The model under review builds one solid part; all positions refer to its coordinate system, in mm. A direction names the side the tool comes from. Round coordinates to 2 decimals unless told otherwise and drop trailing zeros. Write each loop counter-clockwise with the first axis right and the second up, starting at its lowest first coordinate (ties: lowest second). Pieces come first, ordered by that corner, then holes. Notation, with made-up numbers: (46, -40) - (72, -40) arc R14 cw to (72, -21) - close; hole circle Ø6 at (42.5, 66). An arc over 180 degrees is marked (long way). Use one line per item in the form item = value.
Autodesk Inventor part; units mm, degrees
ref_plane "Work Plane1" through (29, 0, 0) normal (0, -1, 0) x (1, 0, 0)
ref_plane "YZ Plane" through (0, 0, 0) normal (1, 0, 0) x (0, 1, 0)
ref_plane "XZ Plane" through (0, 0, 0) normal (0, 1, 0) x (-1, 0, 0)
sketch "Sketch1" plane through (0, 0, 0) normal (0, 0, 1) x (1, 0, 0)
  line L0 (0.2709, 0) -> (19.05, 0)
  line L1 (19.05, 0) -> (19.05, 2.413)
  line L2 (19.05, 2.413) -> (2.1084, 2.413)
  line L3 (2.1084, 2.413) -> (0.0001, 2.413)
  line L4 (0.0001, 2.413) -> (0, 2.413)
  line L5 (0, 2.413) -> (0, 4.5847)
  line L6 (0, 4.5847) -> (-2.5654, 4.5847)
  line L7 (-2.5654, 4.5847) -> (-2.5654, 1.8331)
  line L8 (-2.5654, 1.8331) -> (-0.7874, 1.8331)
  line L9 (-0.7874, 1.8331) -> (0.2709, 0)
  line L10 (-6.8885, 0) -> (23.3731, 0)
  line L11 (0, -0.9169) -> (0, 5.5016)
  line L12 (2.1084, 2.413) -> (0, 2.413) construction
  dimension "d1" = 16.9416
  dimension "d2" = 2.1083
  dimension "d3" = 2.5654
  dimension "d4" = 1.778
  dimension "d5" = 60
  dimension "d6" = 4.826
  dimension "d7" = 4.826
  dimension "d8" = 3.6662
  dimension "d9" = 9.1694
  dimension "d26" = 19.05
revolve "Body" add sketch "Sketch1" angle 360 about axis through (0.2709, 0, 0) along (1, 0, 0) contours L9 L11 L3 L2 L1 L0 | L9 L8 L7 L6 L5 L11
sketch "Sketch2" plane through (-2.5654, 0, 0) normal (-1, 0, 0) x (0, 0, 1)
  circle A0 centre (0, 0) radius 1.8331
  line L0 (0, -6.4186) -> (0, 6.4186)
  line L1 (-6.4186, 0) -> (6.4186, 0)
  line L2 (1.8331, 0) -> (0.9165, -1.5875)
  line L3 (0.9165, -1.5875) -> (-0.9165, -1.5875)
  line L4 (-0.9165, -1.5875) -> (-1.8331, 0)
  line L5 (-1.8331, 0) -> (-0.9165, 1.5875)
  line L6 (-0.9165, 1.5875) -> (0.9165, 1.5875)
  line L7 (0.9165, 1.5875) -> (1.8331, 0)
  point P0 (0, 0)
extrude "Slot" add sketch "Sketch2" against normal up to next contours L7 A0 | A0 L2 | L6 L0 A0 | A0 L0 L3 | L0 L6 A0 | A0 L3 L0 | L4 A0 | A0 L5
fillet "Fillet1" radius 2.3114 1 edges at (-2.5654, -4.5847, 0)
thread "Thread"
chamfer "Chamfer1" distance 0.6492 distance2 0.6492 1 edges at (19.05, -2.413, 0) measured on face at (19.05, -1.2173, -0.6389)
ref_plane "Work Plane1" through (29, 0, 0) normal (0, -1, 0) x (1, 0, 0)
fillet "Fillet2" radius 0.1 1 edges at (0.0001, -2.413, 0)
equation "\"d1\" = GEL"
equation "\"d3\" = KOH"
equation "\"d4\" = INTI"
equation "\"d6\" = GD"
equation "\"d7\" = BDM"
equation "\"d8\" = 1.1547 * SW"
equation "\"d9\" = KOD"
equation "\"d26\" = NLG"
equation "\"d30\" = R"
equation "\"d17\" = RR"
equation "\"d13\" = GEL"
equation "\"d15\" = -0.5 * SPD + 0.5 * GD"
equation "\"d16\" = GUL"
equation "\"GD\" = NND"
equation "\"NLG\" = 19.05"
equation "\"GEL\" = 16.9416"
equation "\"KOD\" = 9.1694"
equation "\"KOH\" = 2.5654"
equation "\"INTI\" = 1.778"
equation "\"GAL\" = 2.1082"
equation "\"GUL\" = 0.64922"
equation "\"BDM\" = NND"
equation "\"SW\" = 3.175"
equation "\"RR\" = 2.3114"
equation "\"SPD\" = 3.52755"
equation "\"R\" = 0.1"
equation "\"TOA\" = 30deg"
equation "\"GD1\" = SPD"
equation "\"THREADDIA\" = 4.826"
equation "\"KOH1\" = 0.508"
equation "\"NND\" = 4.826"
equation "\"E0\" = 3.66725"
properties part number "ANSI B18.3 - 10 - 24 x 3/4" material "Steel, Mild"
(1) To check wall thickness, follow L1, parallel to X at y = -1.5, z = 0.5; L2, parallel to X at y = -1.25, z = 1.25; L3, parallel to Z at x = 13, y = -1.5. State the ranges of each line that lie inside material, in increasing order.
Geometry results:
L1 = -0.64 to 19.05
L2 = -2.57 to 19.05
L3 = -1.89 to 1.89
(2) The part is to be moulded in two halves that separate along Y. For faces 4 (the cylindrical face through (9.122, -1.915, 1.468)), 5 (the flat face through (-1.62, -0.8, -1.37)), 6 (the flat face through (-2.565, -2, 0)), say which applies: +Y half, -Y half, draft (parallel to the pull), parting line (faces both ways), or undercut.
Geometry results:
face_4 = parting line
face_5 = undercut
face_6 = draft
(3) Machinability: for faces 1 (the flat face through (19.05, 0, 0)), 2 (the conical face through (0, -1, 3)), 3 (the flat face through (-2, -1.588, 0)), which of the approach directions +Z, -Z, +X, -X, +Y, -Y give a long, thin tool a straight path to every point of the face, cutting with its end or side? Answer none if there is none.
Geometry results:
face_1 = +Z, -Z, +X, +Y, -Y
face_2 = +X
face_3 = -X
(4) Insertion check: P1, Ø1, axis at x = 0, y = -2, coming from the +Z side; P2, Ø5, axis at x = 7, y = 1.5, coming from the +Z side; P3, Ø1.5, axis at x = 6.5, z = 1, coming from the -Y side. Each pin has a flat end and moves straight along its axis. Give the tip position at first contact, or say it passes through.
Geometry results:
P1 = 4.33
P2 = 2.41
P3 = -2.4
(5) Add section A-A on x = 2.5. Write out the cut boundary in (y, z), then the cut area to 3 significant figures.
Geometry results:
outline = circle Ø4.83 at (0, 0)
area = 18.3 mm2
